```python
from build123d import *

# Parameters (mm, degrees)
EXTRUDE_2_DEPTH     = 5
SKETCH_3_R          = 2.5
CUT_EXTRUDE_2_DEPTH = 15


with BuildPart() as part:
    # 草图2 → 凸台-拉伸2 (new body)
    with BuildSketch(Plane.XY):
        with BuildLine():
            Line((0, 0), (79.999999139, 0))
            ThreePointArc((79.999999139, 0), (85, -4.999999569), (80, -10))
            Line((80, -10), (0, -10))
            ThreePointArc((0, -10), (-5, -5), (0, 0))
        make_face()
    extrude(amount=EXTRUDE_2_DEPTH)

    # 草图3 → 切除-拉伸2 (cut)
    with BuildSketch(Plane.XY.offset(5)):
        with Locations((80, -5)):
            Circle(SKETCH_3_R)
        with BuildLine():
            Line((0, -2.5), (48.378214102, -2.5))
            ThreePointArc((48.378214102, -2.5), (50.878214102, -5), (48.378214102, -7.5))
            Line((48.378214102, -7.5), (0, -7.5))
            ThreePointArc((0, -7.5), (-2.5, -5), (0, -2.5))
        make_face()
    extrude(amount=-CUT_EXTRUDE_2_DEPTH, mode=Mode.SUBTRACT)


solid = part.part
```
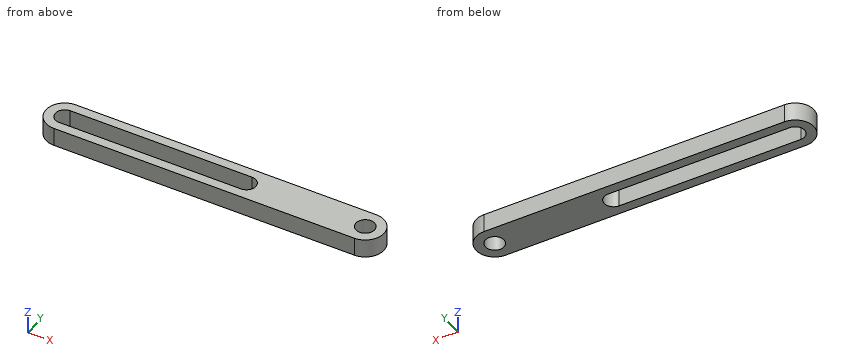
Model file for the job. Use its own axes, mm. Coordinates: 2 decimals unless noted, no trailing zeros. Order: outer loops, then holes, each group sorted by start corner. A loop starts at its lowest first (then second) coordinate and runs counter-clockwise, first axis right, second up. Notation, with made-up numbers: (75.5, 13.25) -> (127.5, 13.25) arc R15 ccw to (127.5, 42.25) -> close; hole circle Ø9 at (61, 66). An arc over 180 degrees is marked (long way). Answer as a JSON object with one key per item and string values. Group by question number.
1) Drill centre lines: L1, parallel to Y at x = 44, z = 1.9; L2, parallel to X at y = -6.5, z = 1.85; L3, parallel to X at y = -5.75, z = 4.05. Where is each one in solid material? Low to high.
2) Cut at C-C, the plane y = -8.75. Write the cut outline in (x, z).
3) Flat gauge pin, fed straight in: pin 1 (4 mm diameter, centred on x = 28.5, y = -7, fed in from +Z). Where does the tip first touch, or does it go through?
4) Cut at B-B, the plane z = 2.9. Write the cut outline in (x, y).
5) Cut at A-A, the plane x = 26.5. Write the cut outline in (y, z), then the cut area to 3 significant figures.
6) Cut at D-D, the plane y = -1.5. Write the cut outline in (x, z), then the cut area to 3 significant figures.
Check values:
{
 "1": {"L1": "y = -10 to -7.5, -2.5 to 0", "L2": "x = -4.77 to -2, 50.38 to 78, 82 to 84.77", "L3": "x = -4.94 to -2.38, 50.76 to 77.62, 82.38 to 84.94"},
 "2": {"outline": "(-3.31, 0) -> (83.31, 0) -> (83.31, 5) -> (-3.31, 5) -> close"},
 "3": {"pin 1": "stops at z = 5"},
 "4": {"outline": "(0, -10) -> (80, -10) arc R5 ccw to (80, 0) -> (0, 0) arc R5 ccw to start; hole (0, -7.5) -> (48.38, -7.5) arc R2.5 ccw to (48.38, -2.5) -> (0, -2.5) arc R2.5 ccw to start; hole circle Ø5 at (80, -5)"},
 "5": {"outline": "(-10, 0) -> (-7.5, 0) -> (-7.5, 5) -> (-10, 5) -> close; (-2.5, 0) -> (0, 0) -> (0, 5) -> (-2.5, 5) -> close", "area": "25.0 mm²"},
 "6": {"outline": "(-3.57, 0) -> (83.57, 0) -> (83.57, 5) -> (-3.57, 5) -> close", "area": "436 mm²"}
}
